Input: dimensioned drawing with shaded views. Units: mm. Origin: part minimum x, y, z. A direction names the side the tool comes from. Coordinates: 2 decimals unless noted, no trailing zeros. Loops run counter-clockwise (first coordinate to the right, second up) from the corner with the lowest first, then second, coordinate; pieces in that order, holes last.
Item 1: Contact query for flat-ended pins moving along their axis: P1, Ø3, axis at x = 5, y = 15, coming from the +Z side; P2, Ø2.5, axis at x = 5, y = 25, coming from the +Z side; P3, Ø12, axis at y = 21.5, z = 63, coming from the +X side; P4, Ø3.5, axis at x = 20, y = 15, coming from the -Z side. Output: stop coordinate, or through.
Item 2: Ray query, line 1 along Y through (x, z) = (5, 56); line 2 along Z through (x, y) = (8, 18.5); line 3 along X through (y, z) = (16.25, 63). Return the intervals inside material, ascending.
Item 3: Pull-direction query (Z, two-part tool) for the marked faces 4, 5 and 6; classes: released by +Z, released by -Z, zero draft, split by the parting line, or undercut.
Item 4: Section D-D on x = 30. Return loops of the section in (y, z).
Item 5: Section A-A on x = 5. Return loops of the section in (y, z).
Item 6: Reachability of the marked faces 1, 2 and 3 from +Z, -Z, +X, -X, +Y, -Y: full face, straight path, thin tool, end or side. Return the list, or none.
Item 7: Section B-B on y = 9.5. Return loops of the section in (x, z), and give its area (3 significant figures).
Item 8: Section C-C on z = 12. Return loops of the section in (x, y).
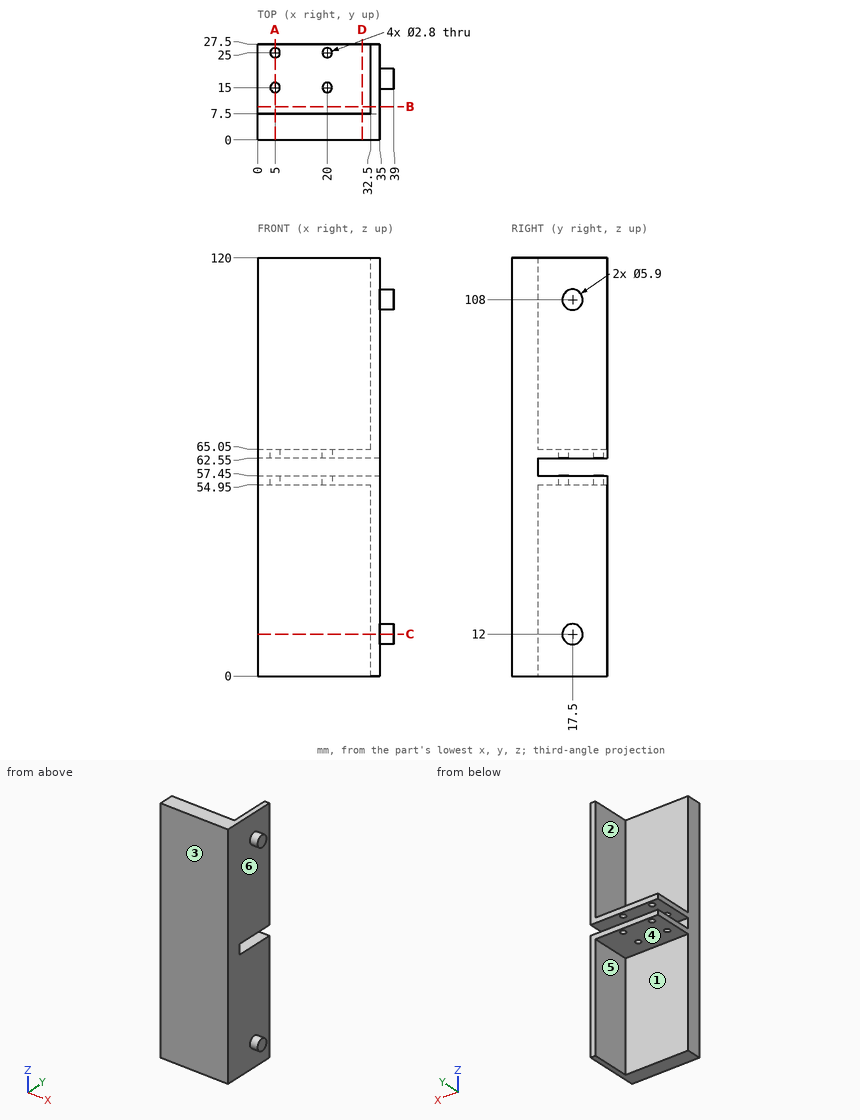
Results found:
1. P1: stops at z = 65.05
1. P2: passes through
1. P3: stops at x = 35
1. P4: stops at z = 54.95
2. line 1: y = 0 to 13.6, 16.4 to 23.6, 26.4 to 27.5
2. line 2: z = 54.95 to 57.45, 62.55 to 65.05
2. line 3: x = 0 to 4.37, 5.63 to 19.37, 20.63 to 35
3. face 4: released by -Z
3. face 5: zero draft
3. face 6: undercut
4. outline: (0, 0) - (7.5, 0) - (7.5, 54.95) - (27.5, 54.95) - (27.5, 57.45) - (7.5, 57.45) - (7.5, 62.55) - (27.5, 62.55) - (27.5, 65.05) - (7.5, 65.05) - (7.5, 120) - (0, 120) - close
5. outline: (0, 0) - (7.5, 0) - (7.5, 54.95) - (13.6, 54.95) - (13.6, 57.45) - (7.5, 57.45) - (7.5, 62.55) - (13.6, 62.55) - (13.6, 65.05) - (7.5, 65.05) - (7.5, 120) - (0, 120) - close; (16.4, 54.95) - (23.6, 54.95) - (23.6, 57.45) - (16.4, 57.45) - close; (16.4, 62.55) - (23.6, 62.55) - (23.6, 65.05) - (16.4, 65.05) - close; (26.4, 54.95) - (27.5, 54.95) - (27.5, 57.45) - (26.4, 57.45) - close; (26.4, 62.55) - (27.5, 62.55) - (27.5, 65.05) - (26.4, 65.05) - close
6. face 1: -Z, -X, +Y
6. face 2: +Z, -X, +Y
6. face 3: +Z, -Z, +X, -X, -Y
7. outline: (0, 54.95) - (32.5, 54.95) - (32.5, 0) - (35, 0) - (35, 57.45) - (0, 57.45) - close; (0, 62.55) - (35, 62.55) - (35, 120) - (32.5, 120) - (32.5, 65.05) - (0, 65.05) - close
7. area: 450 mm2
8. outline: (0, 0) - (35, 0) - (35, 14.55) - (39, 14.55) - (39, 20.45) - (35, 20.45) - (35, 27.5) - (32.5, 27.5) - (32.5, 7.5) - (0, 7.5) - close
